Check sheet for the modelled part. Datum: model origin and axes. Units: mm. Face numbers are marked on the shaded views. A direction names the side the tool comes from. Round coordinates to 2 decimals unless told otherwise and drop trailing zeros. Loops run counter-clockwise (first coordinate to the right, second up) from the corner with the lowest first, then second, coordinate; pieces in that order, holes last. Notation, with made-up numbers: M 75,40 L 80,40 A29 ccw 80,70 Z; hole C -26.75,-10 d8. An arc over 180 degrees is marked long. Write item = value, one per line. Start each with the question number.
(1) Scan lines: L1, parallel to Y at x = 13, z = 9; L2, parallel to X at y = 1.75, z = 22.75; L3, parallel to X at y = 6.25, z = 20 (3 decimals). Record each from-to range of solid material in increasing order. Write a range as from..to.
(2) Set-up check for the marked faces 5, 6, 7, 8 and 9: record each of +Z, -Z, +X, -X, +Y, -Y from which the full face is reachable in a straight line by a thin tool's end or side.
(3) Cross-section at C-C on z = 18.25. Record the boundary of the cut face in (x, y), plus the area to 3 significant figures.
(4) Go/stop test with flat-tipped pins: P1, Ø1.8, axis at y = 2, z = 20.5, coming from the -X side; P2, Ø1, axis at x = 25.5, y = 1, coming from the +Z side; P3, Ø1, axis at x = 18.5, y = 4.5, coming from the -Z side. Record where each tip stops, or that it passes through.
(5) Mould release check, pull along X, two halves, no side actions. Record for the marked faces 1, 2, 3 and 4: pulls with the +X half, pulls with the -X half, needs draft (parallel to the pull), parting line crosses it, or undercut.
(6) Cross-section at A-A on y = 6.75. Record the boundary of the cut face in (x, z) (3 decimals).
(7) Cross-section at D-D on x = -2. Record the boundary of the cut face in (y, z), plus the area to 3 significant figures.
(8) Cross-section at B-B on y = 4.25. Record the boundary of the cut face in (x, z) (3 decimals), plus the area to 3 significant figures.
from build123d import *

# Parameters (mm, degrees)
BOSS_EXTRUDE2_DEPTH = 7.62
CUT_EXTRUDE3_DEPTH  = 2.159
BOSS_EXTRUDE5_DEPTH = 7.62
SKETCH26_R          = 1.4732
CUT_EXTRUDE4_DEPTH  = 28.462559415


with BuildPart() as part:
    # Sketch2 → Boss-Extrude2 (new body)
    with BuildSketch(Plane(origin=(0, 0, 0), x_dir=(1, 0, 0), z_dir=(0, 1, 0))):
        with BuildLine():
            Line((-2.785, -18.89), (-2.785, -22.39))
            Line((-2.785, -22.39), (-9.28719522, -25.422023426))
            Line((-9.28719522, -25.422023426), (-6.46004312, -16.395532832))
            Line((-6.46004312, -16.395532832), (19.152394428, -5.786513834))
            Line((19.152394428, -5.786513834), (27.534185559, -10.170108122))
            Line((27.534185559, -10.170108122), (20.792474901, -12.62389013))
            Line((20.792474901, -12.62389013), (18.317601167, -10.149016395))
            Line((18.317601167, -10.149016395), (16.348308781, -12.118308781))
            Line((16.348308781, -12.118308781), (14.379016395, -14.087601167))
            Line((14.379016395, -14.087601167), (16.85389013, -16.562474901))
            Line((16.85389013, -16.562474901), (14.400108122, -23.304185559))
            ThreePointArc((14.400108122, -23.304185559), (11.890895434, -24.477161025), (9.28719522, -25.422023426))
            Line((9.28719522, -25.422023426), (2.785, -22.39))
            Line((2.785, -22.39), (2.785, -18.89))
            Line((2.785, -18.89), (0, -18.89))
            Line((0, -18.89), (-2.785, -18.89))
        make_face()
    extrude(amount=BOSS_EXTRUDE2_DEPTH)

    # Sketch15 → Cut-Extrude3 (cut)
    with BuildSketch(Plane(origin=(0, 7.62, 0), x_dir=(-1, 0, 0), z_dir=(0, 1, 0))):
        Polygon((-22.217905164, 7.389745786), (7.494030365, 19.696832446), (6.459424884, 16.393558936), (-19.150561514, 5.785555238), align=None)
    extrude(amount=-CUT_EXTRUDE3_DEPTH, mode=Mode.SUBTRACT)

    # Sketch22 → Boss-Extrude5 (add)
    with BuildSketch(Plane(origin=(0, 7.62, 0), x_dir=(1, 0, 0), z_dir=(0, 1, 0))):
        Polygon((-9.28719522, -25.422023426), (-7.494030365, -19.696832446), (-14.565383767, -22.625882929), (-12.740227889, -27.032199003), align=None)
        Polygon((31.114414444, -8.867011376), (27.534185559, -10.170108122), (22.217905164, -7.389745786), (29.289258566, -4.460695302), align=None)
    extrude(amount=-BOSS_EXTRUDE5_DEPTH)

    # Sketch26 → Cut-Extrude4 (cut, through all)
    with BuildSketch(Plane(origin=(8.078449287, 0, 17.324290403), x_dir=(0.9063077870366507, 0, -0.422618261740698), z_dir=(0.422618261740698, 0, 0.9063077870366508))):
        with Locations((-17.478679383, 3.81)):
            Circle(SKETCH26_R)
    cut_extrude4 = extrude(amount=-CUT_EXTRUDE4_DEPTH, mode=Mode.SUBTRACT)

    # Mirror2: Cut-Extrude4 across plane
    add(cut_extrude4.mirror(Plane(origin=(9.626416417, 7.62, 19.01022507), x_dir=(0.38268343236517965, 0, 0.9238795325112495), z_dir=(-0.9238795325112495, 0, 0.38268343236517965))), mode=Mode.SUBTRACT)


solid = part.part
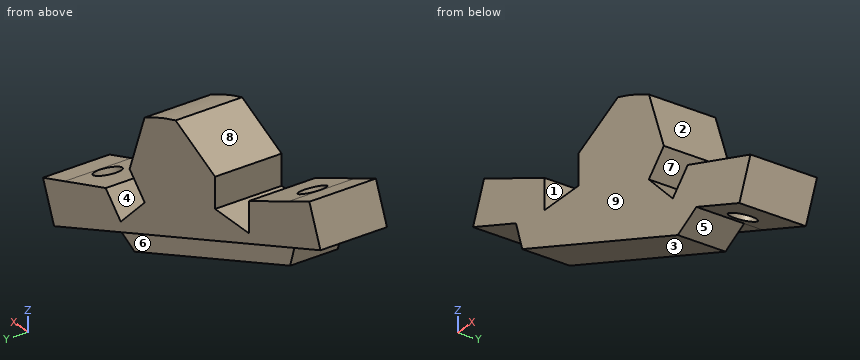
Result:
q1.L1 = 0..5.46
q1.L2 = -14.51..-3.56, 3.56..14.6
q1.L3 = -8.226..-2.785, 2.785..15.603
q2.face_5 = -Z, +Y, -Y
q2.face_6 = -Z, -X, +Y
q2.face_7 = +X, +Y, -Y
q2.face_8 = +Z, +Y, -Y
q2.face_9 = +Z, -Z, +X, -X, -Y
q3.outline = M -7.04,0 L 16.24,0 L 16.24,7.62 L -4,7.62 L -4,5.46 L -7.04,5.46 Z
q3.area = 171 mm^2
q4.P1 = -11.61
q4.P2 = 11.09
q4.P3 = 5.85
q5.face_1 = undercut
q5.face_2 = pulls with the +X half
q5.face_3 = pulls with the -X half
q5.face_4 = undercut
q6.outline = M -14.565,22.626 L 29.289,4.461 L 31.114,8.867 L 20.792,12.624 L 18.318,10.149 L 14.379,14.088 L 16.854,16.562 L 14.4,23.304 A31.072 ccw 9.287,25.422 L 2.785,22.39 L 2.785,18.89 L -2.785,18.89 L -2.785,22.39 L -12.74,27.032 Z
q7.outline = M 0,14.55 L 5.46,14.55 L 5.46,17.42 L 7.62,17.42 L 7.62,18.89 L 0,18.89 Z
q7.area = 26.9 mm^2
q8.outline = M -14.565,22.626 L -10.979,21.14 L -9.037,25.305 L -12.74,27.032 Z; M -8.379,20.063 L -7.494,19.697 L -6.46,16.396 L 19.152,5.787 L 22.218,7.39 L 23.103,7.023 L 24.632,11.226 L 20.792,12.624 L 18.318,10.149 L 14.379,14.088 L 16.854,16.562 L 14.4,23.304 A31.072 ccw 9.287,25.422 L 2.785,22.39 L 2.785,18.89 L -2.785,18.89 L -2.785,22.39 L -6.488,24.117 Z; M 25.703,5.946 L 29.289,4.461 L 31.114,8.867 L 27.275,10.265 Z
q8.area = 323 mm^2
